Work out the finished part from the listing and answer in its coordinate system (mm). Face numbers are marked on the shaded views. A direction names the side the tool comes from. Give positions to 0.01 mm unless a question says otherwise; leave off trailing zeros. Order: outer loops, then holes, each group sorted by start corner. A loop starts at its lowest first (then second) coordinate and runs counter-clockwise, first axis right, second up. Notation, with made-up numbers: (14.25, 62.25) -> (27.25, 62.25) arc R16 ccw to (27.25, 68.25) -> close; hole circle Ø2 at (-5.5, 7.5). An arc over 180 degrees is marked (long way). Use a Markdown table: item, result. Add a question column.
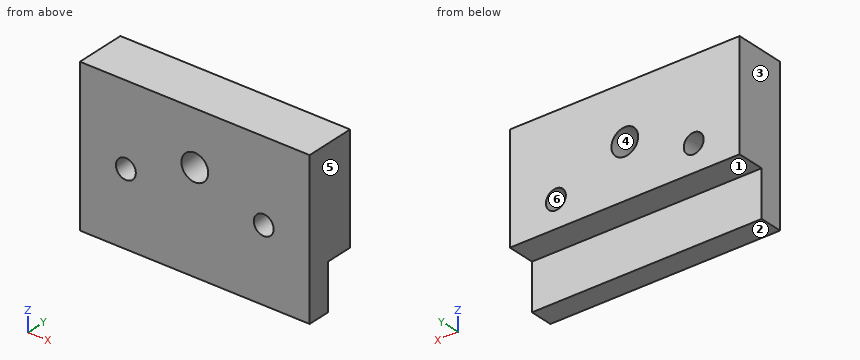
```python
from build123d import *

# Parameters (mm, degrees)
SKETCH_1_W              = 30
SKETCH_1_H              = 20
EXTRUDE_1_DEPTH         = 3
SKETCH_2_W              = 30
SKETCH_2_H              = 14
EXTRUDE_2_DEPTH         = 3.6
HOLE_WIZARD_2_6_2_6_1_D = 2.6
HOLE_WIZARD_3_5_3_5_1_D = 3.5


with BuildPart() as part:
    # 草圖1 → 填料-伸長1 (new body)
    with BuildSketch(Plane(origin=(0, 0, 0), x_dir=(1, 0, 0), z_dir=(0, 1, 0))):
        with Locations((15, 10)):
            Rectangle(SKETCH_1_W, SKETCH_1_H)
    extrude(amount=EXTRUDE_1_DEPTH)

    # 草圖2 → 填料-伸長2 (add)
    with BuildSketch(Plane(origin=(0, 3, 0), x_dir=(1, 0, 0), z_dir=(0, 1, 0))):
        with Locations((15, 7)):
            Rectangle(SKETCH_2_W, SKETCH_2_H)
    extrude(amount=EXTRUDE_2_DEPTH)

    # Ø2.6 (2.6) 直徑孔1 (through all)
    with Locations(Plane(origin=(0, 6.6, 0), x_dir=(1, 0, 0), z_dir=(0, 1, 0))):
        with Locations((6, 10.5), (15, 7), (24, 10.5)):
            Hole(HOLE_WIZARD_2_6_2_6_1_D / 2)

    # Ø3.5 (3.5) 直徑孔1 (through all)
    with Locations(Plane(origin=(0, 6.6, 0), x_dir=(1, 0, 0), z_dir=(0, 1, 0))):
        with Locations((15, 7)):
            Hole(HOLE_WIZARD_3_5_3_5_1_D / 2)


solid = part.part
```
1) Determine the mould class of the marked faces 3, 4, 5 and 6 for opening direction X: released by +X, released by -X, zero draft, split by the parting line, or undercut.
2) The part is cut by section A-A, the plane x = 6. Determine the outline of the cut face in (y, z), then the cut area to 3 significant figures.
3) The part is cut by section D-D, the plane z = -11.5. Determine the outline of the cut face in (x, y).
4) Flat-ended cylindrical pins translate along their axes: pin 1 (1.8 mm diameter, centred on x = 21, y = 4.5, fed in from -Z); pin 2 (5 mm diameter, centred on x = 11.5, z = -18.5, fed in from +Y). Find the tip coordinate at first contact, or state that the pin passes through.
5) The part is cut by section C-C, the plane y = 1. Determine the outline of the cut face in (x, z).
6) Which of the six approach directions +Z, -Z, +X, -X, +Y, -Y give full straight-line access (tool end or side, diameter ignored) to the marked faces 1 and 2?
7) Straight lines are drawn through the part: line 1 (X direction, y = 5.25, z = -10.5); line 2 (X direction, y = 1.75, z = -7); line 3 (Z direction, x = 6, y = 6.5). For each, find the intervals that lie inside material, in ascending order.
8) The part is cut by section B-B, the plane z = -7. Determine the outline of the cut face in (x, y).
A:
| question | item | result |
|---|---|---|
| 1 | face 3 | released by -X |
| 1 | face 4 | undercut |
| 1 | face 5 | released by +X |
| 1 | face 6 | undercut |
| 2 | outline | (0, -20) -> (3, -20) -> (3, -14) -> (6.6, -14) -> (6.6, -11.8) -> (0, -11.8) -> close; (0, -9.2) -> (6.6, -9.2) -> (6.6, 0) -> (0, 0) -> close |
| 2 | area | 93.2 mm^2 |
| 3 | outline | (0, 0) -> (5.17, 0) -> (5.17, 6.6) -> (0, 6.6) -> close; (6.83, 0) -> (23.17, 0) -> (23.17, 6.6) -> (6.83, 6.6) -> close; (24.83, 0) -> (30, 0) -> (30, 6.6) -> (24.83, 6.6) -> close |
| 4 | pin 1 | z = -14 |
| 4 | pin 2 | y = 3 |
| 5 | outline | (0, -20) -> (30, -20) -> (30, 0) -> (0, 0) -> close; hole circle Ø2.6 at (6, -10.5); hole circle Ø3.5 at (15, -7); hole circle Ø2.6 at (24, -10.5) |
| 6 | face 1 | -Z, +X, -X, +Y |
| 6 | face 2 | -Z, +X, -X, +Y, -Y |
| 7 | line 1 | 0 to 4.7, 7.3 to 22.7, 25.3 to 30 |
| 7 | line 2 | 0 to 13.25, 16.75 to 30 |
| 7 | line 3 | -14 to -11.8, -9.2 to 0 |
| 8 | outline | (0, 0) -> (13.25, 0) -> (13.25, 6.6) -> (0, 6.6) -> close; (16.75, 0) -> (30, 0) -> (30, 6.6) -> (16.75, 6.6) -> close |
